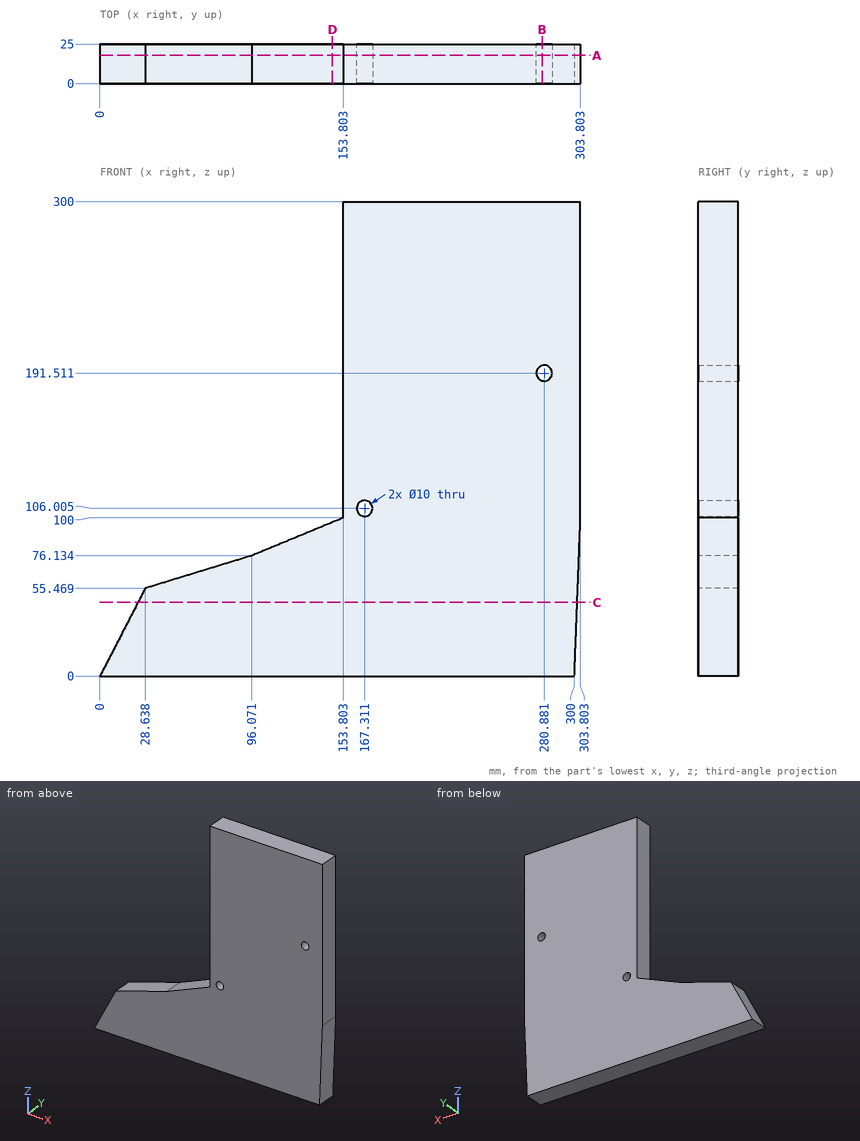
The drawing under review shows one solid part. Ordinate dimensions are in mm from its lowest x, y, z. Coordinates: 2 decimals unless noted, no trailing zeros. Order: outer loops, then holes, each group sorted by start corner. A loop starts at its lowest first (then second) coordinate and runs counter-clockwise, first axis right, second up. Notation, with made-up numbers: (30, 16.25) -> (65, 16.25) arc R21 cw to (65, 31.25) -> close; hole circle Ø5 at (-17.5, 30). An arc over 180 degrees is marked (long way). Answer in a Markdown table with one row per item. Add a question column.
Item 1: We need section A-A on y = 17.75. Write out the cut boundary in (x, z) (1 decimal), plus the area to 3 significant figures.
Item 2: Clearance check with flat-ended pins moving along their axes: pin 1 (12 mm diameter, centred on x = 234.5, z = 47, fed in from -Y); pin 2 (4 mm diameter, centred on y = 21.5, z = 72.5, fed in from +X); pin 3 (12.5 mm diameter, centred on y = 11.5, z = 182.5, fed in from -X); pin 4 (1.5 mm diameter, centred on y = 14.5, z = 74.5, fed in from +X). State where each tip first meets the part, or that it passes through.
Item 3: We need section B-B on x = 279.5. Write out the cut boundary in (y, z) (1 decimal), plus the area to 3 significant figures.
Item 4: We need section D-D on x = 147. Write out the cut boundary in (y, z), plus the area to 3 significant figures.
Item 5: To check wall thickness, follow probe 1 along X at (y, z) = (4, 206); probe 2 along X at (y, z) = (15.5, 110) (1 decimal); probe 3 along Z at (x, y) = (120.5, 20.5). State the ranges of each line that lie inside material, in increasing order.
Item 6: We need section C-C on z = 46.5. Write out the cut boundary in (x, y), plus the area to 3 significant figures.
Final values:
| question | item | result |
|---|---|---|
| 1 | outline | (0, 0) -> (300, 0) -> (303.8, 100) -> (303.8, 300) -> (153.8, 300) -> (153.8, 100) -> (96.1, 76.1) -> (28.6, 55.5) -> close; hole circle Ø10 at (167.3, 106); hole circle Ø10 at (280.9, 191.5) |
| 1 | area | 55,000 mm2 |
| 2 | pin 1 | stops at y = 0 |
| 2 | pin 2 | stops at x = 302.83 |
| 2 | pin 3 | stops at x = 153.8 |
| 2 | pin 4 | stops at x = 302.86 |
| 3 | outline | (0, 0) -> (25, 0) -> (25, 186.7) -> (0, 186.7) -> close; (0, 196.3) -> (25, 196.3) -> (25, 300) -> (0, 300) -> close |
| 3 | area | 7,260 mm2 |
| 4 | outline | (0, 0) -> (25, 0) -> (25, 97.19) -> (0, 97.19) -> close |
| 4 | area | 2,430 mm2 |
| 5 | probe 1 | x = 153.8 to 303.8 |
| 5 | probe 2 | x = 153.8 to 164.3, 170.3 to 303.8 |
| 5 | probe 3 | z = 0 to 86.23 |
| 6 | outline | (24.01, 0) -> (301.77, 0) -> (301.77, 25) -> (24.01, 25) -> close |
| 6 | area | 6,940 mm2 |
